Design review of the part built by this model. Coordinates are the model's own, in mm. Give positions to 0.01 mm unless a question says otherwise; leave off trailing zeros. Loops run counter-clockwise (first coordinate to the right, second up) from the corner with the lowest first, then second, coordinate; pieces in that order, holes last. Notation, with made-up numbers: (81.5, 54) -> (127.5, 54) arc R30 ccw to (127.5, 85) -> close; hole circle Ø11 at (66.5, -34.5). An arc over 180 degrees is marked (long way). Answer in a Markdown table with one row per item. Add a question column.
(1) Consider section C-C on x = 43. Write out the cut boundary in (y, z).
(2) For line 1 (X direction, y = 1.3, z = -3.5); line 2 (X direction, y = 1.3, z = -41.5); line 3 (Z direction, x = 21, y = 0.55), list the stretches that pass through material, from the lowest coordinate up.
(3) Consider section A-A on z = -3.5. Write out the cut boundary in (x, y), then the cut area to 3 significant figures.
(4) Consider section D-D on z = -46.5. Write out the cut boundary in (x, y), then the cut area to 3 significant figures.
(5) For pin 1 (2.5 mm diameter, centred on x = 8, z = -3.5, fed in from -Y), flat-tipped, find the tip position at first contact; note if it passes through.
(6) Consider section B-B on y = 1.55. Write out the cut boundary in (x, z), then the cut area to 3 significant figures.
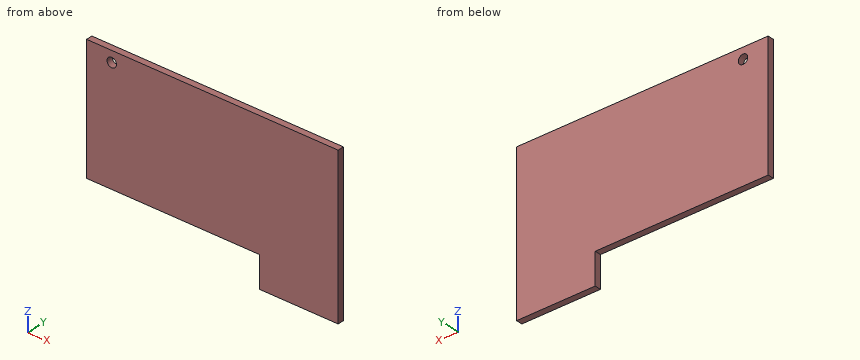
from build123d import *

# Parameters (mm, degrees)
SKETCH1_W           = 80
SKETCH1_H           = 50
BOSS_EXTRUDE1_DEPTH = 2
SKETCH2_R           = 1.5
CUT_EXTRUDE1_DEPTH  = 2
SKETCH3_W           = 55
SKETCH3_H           = 10
CUT_EXTRUDE2_DEPTH  = 95.361008897


with BuildPart() as part:
    # Sketch1 → Boss-Extrude1 (new body)
    with BuildSketch(Plane(origin=(0, 0, 0), x_dir=(1, 0, 0), z_dir=(0, 1, 0))):
        with Locations((40, 25)):
            Rectangle(SKETCH1_W, SKETCH1_H)
    extrude(amount=BOSS_EXTRUDE1_DEPTH)

    # Sketch2 → Cut-Extrude1 (cut)
    with BuildSketch(Plane(origin=(0, 2, 0), x_dir=(1, 0, 0), z_dir=(0, 1, 0))):
        with Locations(Location((8, 3.5, 0), (0, 0, 270))):
            Circle(SKETCH2_R)
    extrude(amount=-CUT_EXTRUDE1_DEPTH, mode=Mode.SUBTRACT)

    # Sketch3 → Cut-Extrude2 (cut, through all)
    with BuildSketch(Plane(origin=(0, 2, 0), x_dir=(1, 0, 0), z_dir=(0, 1, 0))):
        with Locations((27.5, 45)):
            Rectangle(SKETCH3_W, SKETCH3_H)
    extrude(amount=-CUT_EXTRUDE2_DEPTH, mode=Mode.SUBTRACT)


solid = part.part
Values follow:
| question | item | result |
|---|---|---|
| 1 | outline | (0, -40) -> (2, -40) -> (2, 0) -> (0, 0) -> close |
| 2 | line 1 | 0 to 6.5, 9.5 to 80 |
| 2 | line 2 | 55 to 80 |
| 2 | line 3 | -40 to 0 |
| 3 | outline | (0, 0) -> (6.5, 0) -> (6.5, 2) -> (0, 2) -> close; (9.5, 0) -> (80, 0) -> (80, 2) -> (9.5, 2) -> close |
| 3 | area | 154 mm2 |
| 4 | outline | (55, 0) -> (80, 0) -> (80, 2) -> (55, 2) -> close |
| 4 | area | 50.0 mm2 |
| 5 | pin 1 | through |
| 6 | outline | (0, -40) -> (55, -40) -> (55, -50) -> (80, -50) -> (80, 0) -> (0, 0) -> close; hole circle Ø3 at (8, -3.5) |
| 6 | area | 3,440 mm2 |
